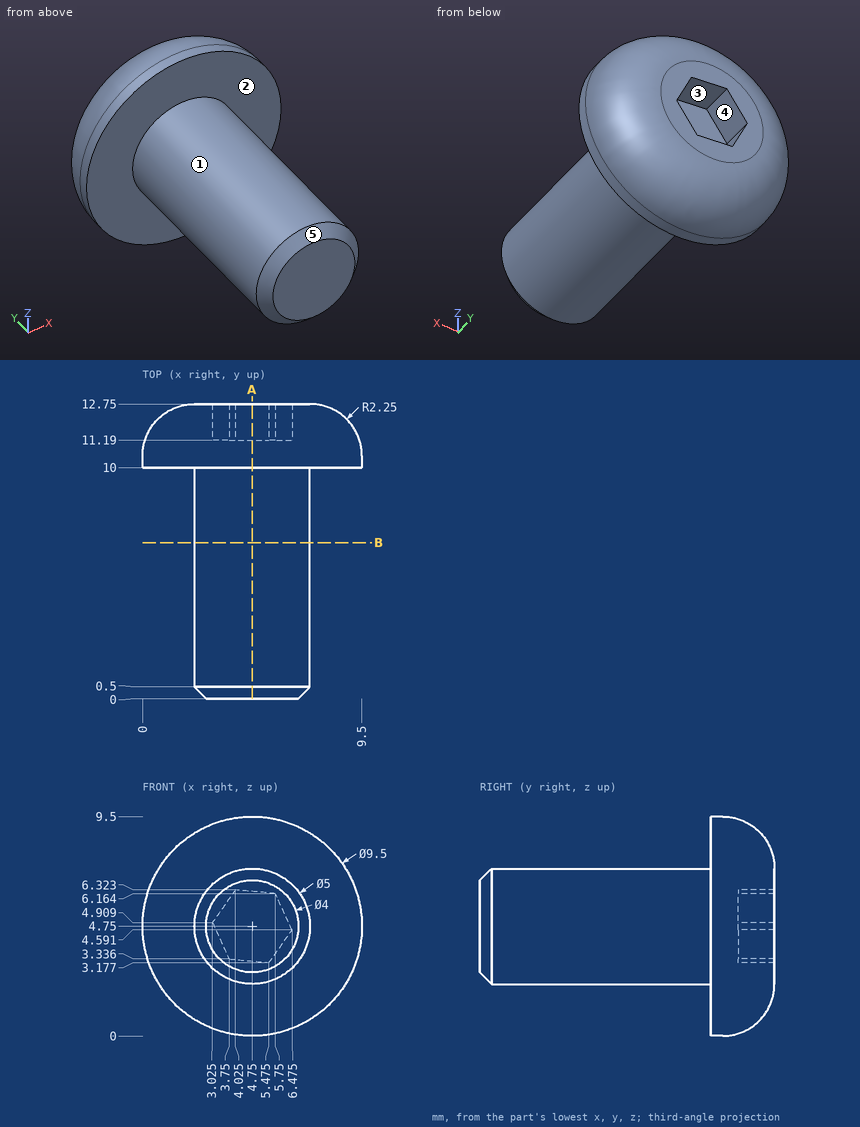
Can you work these out from the drawing? Everything is in mm from the part's minimum corner. A direction names the side the tool comes from. Coordinates: 2 decimals unless noted, no trailing zeros. Loops run counter-clockwise (first coordinate to the right, second up) from the corner with the lowest first, then second, coordinate; pieces in that order, holes last. Notation, with made-up numbers: M -12,48 L 22,48 A19 cw 22,68 Z; hole C 73,70 d4. An arc over 180 degrees is marked long. One line per item, written item: value.
1. Thinking about a two-plate mould opening in X: for the marked faces 1, 2 and 3, which applies, +X half, -X half, draft (parallel to the pull), parting line (faces both ways), or undercut?
Geometry says:
face 1: parting line
face 2: draft
face 3: undercut
2. Please list where these lines run through material, in increasing order: probe 1 along Z at (x, y) = (4.75, 5.5); probe 2 along Y at (x, z) = (4.25, 0.75); probe 3 along Z at (x, y) = (2.5, 6.25).
Geometry says:
probe 1: z = 2.25 to 7.25
probe 2: y = 10 to 12.15
probe 3: z = 3.66 to 5.84
3. Will these pins go through, and if not, where does the flat tip stop? pin 1 Ø1 at (x, z) = (3.5, 4) entering from -Y; pin 2 Ø1 at (y, z) = (4, 1) entering from -X; pin 3 Ø1 at (y, z) = (9, 4.5) entering from -X; pin 4 Ø3 at (x, y) = (7.5, 11) entering from +Z.
Geometry says:
pin 1: stops at y = 0
pin 2: passes through
pin 3: stops at x = 2.25
pin 4: stops at z = 9.32
4. Imagine slicing it at B-B (y = 6.75). List the corners of the cut face in (x, z) for me, and give its area (3 significant figures).
Geometry says:
outline: C 4.75,4.75 d5
area: 19.6 mm2
5. On a 3-axis mill with a long thin cutter (end or side, diameter ignored), from which of +Z, -Z, +X, -X, +Y, -Y can I reach the whole of each face in a straight line? I mean the marked faces 4 and 5. Say none if no direction works.
Geometry says:
face 4: +Y
face 5: -Y
6. Imagine slicing it at A-A (x = 4.75). List the corners of the cut face in (y, z) for me.
Geometry says:
outline: M 0,2.75 L 0.5,2.25 L 10,2.25 L 10,0 L 10.5,0 A2.25 ccw 12.75,2.25 L 12.75,3.24 L 11.19,3.24 L 11.19,6.26 L 12.75,6.26 L 12.75,7.25 A2.25 ccw 10.5,9.5 L 10,9.5 L 10,7.25 L 0.5,7.25 L 0,6.75 Z
